Model file for the job. Use its own axes, mm. A direction names the side the tool comes from. Round coordinates to 2 decimals unless told otherwise and drop trailing zeros. Order: outer loops, then holes, each group sorted by start corner. A loop starts at its lowest first (then second) coordinate and runs counter-clockwise, first axis right, second up. Notation, with made-up numbers: (16.5, 80) - (70.5, 80) arc R16 ccw to (70.5, 109) - close; hole circle Ø4 at (-35, 28.5). An arc over 180 degrees is marked (long way). Write item = value, one per line.
```python
from build123d import *

# Parameters (mm, degrees)
SKETCH_1_R          = 12
SKETCH_1_R_2        = 4.5
EXTRUDE_1_DEPTH     = 7
SKETCH_2_R          = 13.5
SKETCH_2_R_2        = 4.5
EXTRUDE_2_DEPTH     = 1.5
SKETCH_3_R          = 10.5
SKETCH_3_R_2        = 6.25
CUT_EXTRUDE_1_DEPTH = 0.3
SKETCH_4_R          = 10.5
SKETCH_4_R_2        = 6.25
CUT_EXTRUDE_2_DEPTH = 0.3


with BuildPart() as part:
    # 草图1 → 凸台-拉伸1 (new body)
    with BuildSketch(Plane(origin=(0, 0, 0), x_dir=(1, 0, 0), z_dir=(0, 1, 0))):
        Circle(SKETCH_1_R)
        Circle(SKETCH_1_R_2, mode=Mode.SUBTRACT)
    extrude(amount=EXTRUDE_1_DEPTH)

    # 草图2 → 凸台-拉伸2 (add)
    with BuildSketch(Plane.XZ):
        Circle(SKETCH_2_R)
        Circle(SKETCH_2_R_2, mode=Mode.SUBTRACT)
    extrude(amount=EXTRUDE_2_DEPTH)

    # 草图3 → 切除-拉伸1 (cut)
    with BuildSketch(Plane(origin=(0, 7, 0), x_dir=(1, 0, 0), z_dir=(0, 1, 0))):
        with Locations((0, 0.185580925)):
            Circle(SKETCH_3_R)
        Circle(SKETCH_3_R_2, mode=Mode.SUBTRACT)
    extrude(amount=-CUT_EXTRUDE_1_DEPTH, mode=Mode.SUBTRACT)

    # 草图4 → 切除-拉伸2 (cut)
    with BuildSketch(Plane.XZ.offset(1.5)):
        Circle(SKETCH_4_R)
        Circle(SKETCH_4_R_2, mode=Mode.SUBTRACT)
    extrude(amount=-CUT_EXTRUDE_2_DEPTH, mode=Mode.SUBTRACT)


solid = part.part
```
1) 3-axis set-ups, long thin cutter, end or side, ignore diameter. For faces 4 (the face through (-1.37, -1.35, 10.41)), 5 (the face through (5.96, 6.85, -1.88)), 6 (the face through (0, -1.5, -11)): which of +Z, -Z, +X, -X, +Y, -Y reach the whole face in a straight line?
Conclusion:
face_4 = -Y
face_5 = +Y
face_6 = +Z, -Z, +X, -X, -Y
2) Cut at D-D (x = 8). Write the cut outline in (y, z), and give its area (3 significant figures).
Conclusion:
outline = (-1.5, -10.87) - (0, -10.87) - (0, -8.94) - (7, -8.94) - (7, -6.99) - (6.7, -6.99) - (6.7, 6.62) - (7, 6.62) - (7, 8.94) - (0, 8.94) - (0, 10.87) - (-1.5, 10.87) - (-1.5, 6.8) - (-1.2, 6.8) - (-1.2, -6.8) - (-1.5, -6.8) - close
area = 150 mm^2
3) Cut at B-B (z = 9.75). Write the cut outline in (x, y), and give its area (3 significant figures).
Conclusion:
outline = (-9.34, -1.5) - (-3.9, -1.5) - (-3.9, -1.2) - (3.9, -1.2) - (3.9, -1.5) - (9.34, -1.5) - (9.34, 0) - (7, 0) - (7, 7) - (3.4, 7) - (3.4, 6.7) - (-3.4, 6.7) - (-3.4, 7) - (-7, 7) - (-7, 0) - (-9.34, 0) - close
area = 122 mm^2
4) Cut at C-C (y = 2). Write the cut outline in (x, z), and give its area (3 significant figures).
Conclusion:
outline = circle Ø24 at (0, 0); hole circle Ø9 at (0, 0)
area = 389 mm^2
5) Wall check: line 1 along Z through (x, y) = (0, 6.85); line 2 along X through (y, z) = (3.75, 0). Give the ranges that are in metal, low to high.
Conclusion:
line_1 = -12 to -10.69, -6.25 to -4.5, 4.5 to 6.25, 10.31 to 12
line_2 = -12 to -4.5, 4.5 to 12
6) Cut at A-A (x = 0). Write the cut outline in (y, z), and give its area (3 significant figures).
Conclusion:
outline = (-1.5, -13.5) - (0, -13.5) - (0, -12) - (7, -12) - (7, -10.69) - (6.7, -10.69) - (6.7, -6.25) - (7, -6.25) - (7, -4.5) - (-1.5, -4.5) - (-1.5, -6.25) - (-1.2, -6.25) - (-1.2, -10.5) - (-1.5, -10.5) - close; (-1.5, 4.5) - (7, 4.5) - (7, 6.25) - (6.7, 6.25) - (6.7, 10.31) - (7, 10.31) - (7, 12) - (0, 12) - (0, 13.5) - (-1.5, 13.5) - (-1.5, 10.5) - (-1.2, 10.5) - (-1.2, 6.25) - (-1.5, 6.25) - close
area = 127 mm^2
7) Flat gauge pins, fed straight in: pin 1 Ø6.5 at (x, z) = (-2, 0) entering from +Y; pin 2 Ø4 at (x, y) = (-10, 2.5) entering from -Z; pin 3 Ø4 at (y, z) = (1, -10.5) entering from +X; pin 4 Ø1 at (x, y) = (3.5, 6) entering from -Z. Where does each tip first touch, or does it go through?
Conclusion:
pin_1 = 7
pin_2 = -8.94
pin_3 = 10.27
pin_4 = -11.62
8) Mould opens along X. For faces 1 (the face through (-0.59, 2.81, 4.46)), 2 (the face through (3, 7, 4)), 3 (the face through (-2.93, -0.74, -13.18)) say: +X half, -X half, draft (parallel to the pull), parting line (faces both ways), or undercut.
Conclusion:
face_1 = undercut
face_2 = draft
face_3 = parting line
